from build123d import *

# Parameters (mm, degrees)
SKETCH_1_W          = 15
SKETCH_1_H          = 50
SKETCH_1_R          = 1.65
EXTRUDE_1_DEPTH     = 15
SKETCH_2_R          = 1.65
CUT_EXTRUDE_1_DEPTH = 15
FILLET_1_R          = 2


with BuildPart() as part:
    # ｽｹｯﾁ1 → ﾎﾞｽ - 押し出し1 (new body)
    with BuildSketch(Plane.XY):
        with Locations((7.5, 25)):
            Rectangle(SKETCH_1_W, SKETCH_1_H)
        with Locations((5.5, 5)):
            Circle(SKETCH_1_R, mode=Mode.SUBTRACT)
        with Locations(Location((5.5, 45, 0), (0, 0, 180))):
            Circle(SKETCH_1_R, mode=Mode.SUBTRACT)
    extrude(amount=EXTRUDE_1_DEPTH)

    # ｽｹｯﾁ2 → ｶｯﾄ - 押し出し1 (cut)
    with BuildSketch(Plane.ZY):
        with Locations((7.5, 40)):
            Circle(SKETCH_2_R)
        with Locations((7.5, 10)):
            Circle(SKETCH_2_R)
    extrude(amount=-CUT_EXTRUDE_1_DEPTH, mode=Mode.SUBTRACT)

    # ﾌｨﾚｯﾄ1
    fillet_1_edges = [part.edges().sort_by_distance(p)[0] for p in [
        (0, 50, 7.5),
        (15, 50, 7.5),
        (15, 0, 7.5),
        (0, 0, 7.5),
    ]]
    fillet(fillet_1_edges, radius=FILLET_1_R)


solid = part.part
Source: CAD feature listing. Evaluate the final solid. Frame: model axes, mm. Coordinates: 2 decimals unless noted, no trailing zeros. Loops run counter-clockwise (first coordinate to the right, second up) from the corner with the lowest first, then second, coordinate; pieces in that order, holes last. Notation, with made-up numbers: (50.5, 40.25) -> (96.5, 40.25) arc R32 ccw to (96.5, 74.25) -> close; hole circle Ø9 at (23.25, 79.25). An arc over 180 degrees is marked (long way). Answer in a Markdown table with one row per item. Add a question column.
Q1. Ray query, line 1 along Y through (x, z) = (10.25, 7.5); line 2 along X through (y, z) = (45, 4); line 3 along Y through (x, z) = (4.5, 3.75). Return the intervals inside material, ascending.
Q2. Section D-D on x = 10.5. Return the cut outline in (y, z).
Q3. Section C-C on y = 45. Return the cut outline in (x, z), and give its area (4 significant figures).
Q4. Section B-B on z = 7.25. Return the cut outline in (x, y).
Q5. Pull-direction query (Y, two-part tool) for faces 1 (the face through (0.57, 49.4, 7.6)), 2 (the face through (5.715, 43.364, 7.395)), 3 (the face through (14.4, 0.57, 7.6)), 4 (the face through (15, 25, 7)); classes: pulls with the +Y half, pulls with the -Y half, needs draft (parallel to the pull), parting line crosses it, or undercut.
Q6. Section A-A on x = 5.5. Return the cut outline in (y, z).
Computed values:
| question | item | result |
|---|---|---|
| 1 | line 1 | y = 0 to 8.35, 11.65 to 38.35, 41.65 to 50 |
| 1 | line 2 | x = 0 to 3.85, 7.15 to 15 |
| 1 | line 3 | y = 0 to 3.69, 6.31 to 43.69, 46.31 to 50 |
| 2 | outline | (0, 0) -> (50, 0) -> (50, 15) -> (0, 15) -> close; hole circle Ø3.3 at (10, 7.5); hole circle Ø3.3 at (40, 7.5) |
| 3 | outline | (0, 0) -> (3.85, 0) -> (3.85, 15) -> (0, 15) -> close; (7.15, 0) -> (15, 0) -> (15, 15) -> (7.15, 15) -> close |
| 3 | area | 175.5 mm^2 |
| 4 | outline | (0, 2) arc R2 ccw to (2, 0) -> (13, 0) arc R2 ccw to (15, 2) -> (15, 8.37) -> (0, 8.37) -> close; (0, 11.63) -> (15, 11.63) -> (15, 38.37) -> (0, 38.37) -> close; (0, 41.63) -> (15, 41.63) -> (15, 48) arc R2 ccw to (13, 50) -> (2, 50) arc R2 ccw to (0, 48) -> close; hole circle Ø3.3 at (5.5, 5); hole circle Ø3.3 at (5.5, 45) |
| 5 | face 1 | pulls with the +Y half |
| 5 | face 2 | undercut |
| 5 | face 3 | pulls with the -Y half |
| 5 | face 4 | needs draft |
| 6 | outline | (0, 0) -> (3.35, 0) -> (3.35, 15) -> (0, 15) -> close; (6.65, 0) -> (43.35, 0) -> (43.35, 15) -> (6.65, 15) -> close; (46.65, 0) -> (50, 0) -> (50, 15) -> (46.65, 15) -> close; hole circle Ø3.3 at (10, 7.5); hole circle Ø3.3 at (40, 7.5) |
